Check sheet for the modelled part. Datum: model origin and axes. Units: mm. A direction names the side the tool comes from. Round coordinates to 2 decimals unless told otherwise and drop trailing zeros. Order: outer loops, then holes, each group sorted by start corner. A loop starts at its lowest first (then second) coordinate and runs counter-clockwise, first axis right, second up. Notation, with made-up numbers: (80, 19) -> (131, 19) arc R22 ccw to (131, 36) -> close; hole circle Ø7 at (46.25, 13). An arc over 180 degrees is marked (long way). Answer in a Markdown table with one row per item. Add a question column.
1. Sectioned sample at A-A, the plane y = -7.5. Record the boundary of the cut face in (x, z), then the cut area to 3 significant figures.
2. Material ranges on L1, parallel to Y at x = 7.6, z = 2.5; L2, parallel to Y at x = 7, z = 0.8; L3, parallel to Y at x = 1.8, z = 2.5, recorded low to high. Write a range as from..to.
3. Sectioned sample at C-C, the plane x = 4.75. Record the boundary of the cut face in (y, z), then the cut area to 3 significant figures.
4. Draft check along Y on faces 4 (the cylindrical face through (1.75, -0.04, 4.21)), 5 (the flat face through (10, 0, 2)), 6 (the flat face through (5, 10, 2)). Enter one of: +Y half, -Y half, draft (parallel to the pull), parting line (faces both ways), or undercut.
5. Access from +Z, -Z, +X, -X, +Y, -Y to the whole of each face (thin tool, end or side, straight path). Record for faces 1 (the flat face through (6, 8, 1)), 2 (the flat face through (2, 0, 1.6)), 3 (the flat face through (0, 6, 2)).
6. Depth check by flat-ended pin: P1, Ø3, axis at y = 7.5, z = 2.5, coming from the +X side; P2, Ø0.5, axis at y = 0.5, z = 2.5, coming from the -X side. Enter the tip coordinate at first touch or a pass-through.
7. Sectioned sample at D-D, the plane y = 0. Record the boundary of the cut face in (x, z).
8. Sectioned sample at B-B, the plane z = 2.5. Record the boundary of the cut face in (x, y), then the cut area to 3 significant figures.
Autodesk Inventor part; units mm, degrees
ref_plane "YZ Plane" through (0, 0, 0) normal (1, 0, 0) x (0, 1, 0)
ref_plane "XZ Plane" through (0, 0, 0) normal (0, 1, 0) x (-1, 0, 0)
ref_plane "XY Plane" through (0, 0, 0) normal (0, 0, 1) x (1, 0, 0)
sketch "Sketch1" plane through (0, 0, 0) normal (0, 0, 1) x (1, 0, 0)
  line L0 (10, -10) -> (-10, -10)
  line L1 (-10, -10) -> (-10, 10)
  line L2 (-10, 10) -> (10, 10)
  line L3 (10, 10) -> (10, -10)
  line L4 (10, -10) -> (-10, 10) construction
  line L5 (-10, -10) -> (10, 10) construction
  line L6 (10, -10) -> (6, -10)
  line L7 (6, 10) -> (10, 10)
  line L8 (10, 10) -> (10, -10)
  line L9 (0, 10) -> (0, -10)
  line L10 (0, -10) -> (0, 10)
  point P0 (0, 0)
  dimension "d0" = 20
  dimension "d1" = 20
extrude "Extrusion1" add sketch "Sketch1" along normal blind 5 contours L0 L9 L2 L3
ref_plane "Work Plane1" through (0, 0, 2.5) normal (0, 0, 1) x (1, 0, 0)
sketch "Sketch2" plane through (0, 0, 2.5) normal (0, 0, 1) x (1, 0, 0)
  line L0 (0, 10) -> (0, -10)
  line L1 (0, 3.1754) -> (2.75, 1.5877)
  line L2 (2.75, 1.5877) -> (2.75, -1.5877)
  line L3 (2.75, -1.5877) -> (0, -3.1754)
  line L4 (0, -3.1754) -> (-2.75, -1.5877)
  line L5 (-2.75, -1.5877) -> (-2.75, 1.5877)
  line L6 (-2.75, 1.5877) -> (0, 3.1754)
  point P0 (0, 0)
  point P1 (0, 0)
  dimension "d12" = 5.5
extrude "Extrusion2" cut sketch "Sketch2" along normal mid plane 1.8
sketch "Sketch3" plane through (0, 0, 5) normal (0, 0, 1) x (1, 0, 0)
  circle A0 centre (0, 0) radius 1.75
  dimension "d15" = 3.5
extrude "Extrusion3" cut sketch "Sketch3" against normal blind 8
sketch "Sketch4" plane through (10, -10, 0) normal (1, 0, 0) x (0, 0, -1)
  circle A0 centre (-2.5, 17.5) radius 1.3
  circle A1 centre (-2.5, 2.5) radius 1.3
  line L0 (0, 20) -> (-5, 20)
  line L1 (0, 0) -> (-5, 0)
  line L2 (0, 0) -> (0, 20)
  point P0 (0, 10)
  dimension "d18" = 2.5
  dimension "d19" = 2.5
  dimension "d20" = 2.5
  dimension "d21" = 2.5
  dimension "d22" = 2.6
  dimension "d23" = 2.6
extrude "Extrusion4" cut sketch "Sketch4" against normal blind 25
sketch "Sketch5" plane through (10, -10, 0) normal (1, 0, 0) x (0, 0, -1)
  circle A0 centre (-2.5, 17.5) radius 1.3
  circle A1 centre (-2.5, 17.5) radius 2
  circle A2 centre (-2.5, 2.5) radius 1.3
  circle A3 centre (-2.5, 2.5) radius 2
  point P0 (0, 10)
  dimension "d26" = 4
  dimension "d27" = 4
extrude "Extrusion5" cut sketch "Sketch5" against normal blind 4 contours A0 | A1 | A2 | A3
equation "\"d18\" = d19"
equation "\"d20\" = d19"
equation "\"d21\" = d19"
equation "\"d23\" = d22"
equation "\"d27\" = d26"
properties part number "POMSliderMotor"
Answer key:
| question | item | result |
|---|---|---|
| 1 | outline | (0, 0) -> (10, 0) -> (10, 0.5) -> (6, 0.5) -> (6, 1.2) -> (0, 1.2) -> close; (0, 3.8) -> (6, 3.8) -> (6, 4.5) -> (10, 4.5) -> (10, 5) -> (0, 5) -> close |
| 1 | area | 18.4 mm² |
| 2 | L1 | y = -10..-9.5, -5.5..5.5, 9.5..10 |
| 2 | L2 | y = -10..-8.55, -6.45..6.45, 8.55..10 |
| 2 | L3 | y = -10..-8.8, -6.2..-2.14, 2.14..6.2, 8.8..10 |
| 3 | outline | (-10, 0) -> (10, 0) -> (10, 5) -> (-10, 5) -> close; hole circle Ø2.6 at (-7.5, 2.5); hole circle Ø2.6 at (7.5, 2.5) |
| 3 | area | 89.4 mm² |
| 4 | face 4 | undercut |
| 4 | face 5 | draft |
| 4 | face 6 | +Y half |
| 5 | face 1 | +X |
| 5 | face 2 | -X |
| 5 | face 3 | +Z, -Z, -X, +Y, -Y |
| 6 | P1 | stops at x = 6 |
| 6 | P2 | stops at x = 2.75 |
| 7 | outline | (1.75, 0) -> (10, 0) -> (10, 5) -> (1.75, 5) -> (1.75, 3.4) -> (2.75, 3.4) -> (2.75, 1.6) -> (1.75, 1.6) -> close |
| 8 | outline | (0, -10) -> (10, -10) -> (10, -9.5) -> (6, -9.5) -> (6, -8.8) -> (0, -8.8) -> close; (0, -6.2) -> (6, -6.2) -> (6, -5.5) -> (10, -5.5) -> (10, 5.5) -> (6, 5.5) -> (6, 6.2) -> (0, 6.2) -> (0, 3.18) -> (2.75, 1.59) -> (2.75, -1.59) -> (0, -3.18) -> close; (0, 8.8) -> (6, 8.8) -> (6, 9.5) -> (10, 9.5) -> (10, 10) -> (0, 10) -> close |
| 8 | area | 124 mm² |
